Could you check a few things on this model? Use its own coordinates, in mm. Face numbers are marked on the shaded views. Give positions to 0.01 mm unless a question says otherwise; leave off trailing zeros. Order: outer loops, then holes, each group sorted by start corner. A loop starts at its lowest first (then second) coordinate and runs counter-clockwise, first axis right, second up. Notation, with made-up numbers: (-35.75, -13.5) -> (8.25, -13.5) arc R29 cw to (8.25, 8.5) -> close; hole circle Ø3 at (-22, 6.25). An arc over 180 degrees is marked (long way). One line per item, written item: value.
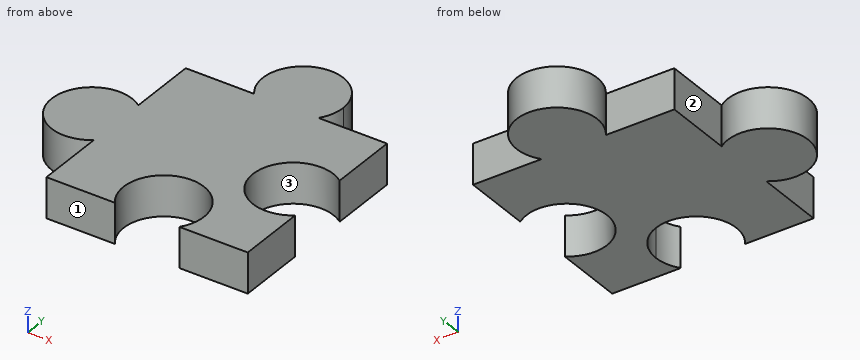
```python
from build123d import *

# Parameters (mm, degrees)
F1_DEPTH = 2.54


with BuildPart() as f1:
    # F0 (on Top) → F1 (new body)
    with BuildSketch(Plane.XY):
        with BuildLine():
            Line((-49.9644750565, 16.7031875085), (-49.9644750565, 20.7671875085))
            ThreePointArc((-49.9644750565, 20.7671875085), (-54.0284750565, 18.7351875085), (-49.9644750565, 16.7031875085))
        make_face()
        with BuildLine():
            ThreePointArc((-48.9484750565, 18.7351875085), (-49.2166299914, 19.8711100411), (-49.9644750565, 20.7671875085))
            Line((-49.9644750565, 20.7671875085), (-49.9644750565, 16.7031875085))
            ThreePointArc((-49.9644750565, 16.7031875085), (-49.2166299914, 17.599264976), (-48.9484750565, 18.7351875085))
        make_face()
        with BuildLine():
            Line((-45.6464750565, 25.0851875085), (-49.9644750565, 25.0851875085))
            Line((-49.9644750565, 25.0851875085), (-49.9644750565, 20.7671875085))
            ThreePointArc((-49.9644750565, 20.7671875085), (-49.2166299914, 19.8711100411), (-48.9484750565, 18.7351875085))
            ThreePointArc((-48.9484750565, 18.7351875085), (-49.2166299914, 17.599264976), (-49.9644750565, 16.7031875085))
            Line((-49.9644750565, 16.7031875085), (-49.9644750565, 12.3851875085))
            Line((-49.9644750565, 12.3851875085), (-45.6464750565, 12.3851875085))
            ThreePointArc((-45.6464750565, 12.3851875085), (-44.4176935822, 16.3188430856), (-41.0744750565, 13.9091875085))
            ThreePointArc((-41.0744750565, 13.9091875085), (-41.2048194795, 13.1059689828), (-41.5824750565, 12.3851875085))
            Line((-41.5824750565, 12.3851875085), (-37.2644750565, 12.3851875085))
            Line((-37.2644750565, 12.3851875085), (-37.2644750565, 16.7031875085))
            ThreePointArc((-37.2644750565, 16.7031875085), (-41.3284750565, 18.7351875085), (-37.2644750565, 20.7671875085))
            Line((-37.2644750565, 20.7671875085), (-37.2644750565, 25.0851875085))
            Line((-37.2644750565, 25.0851875085), (-41.5824750565, 25.0851875085))
            ThreePointArc((-41.5824750565, 25.0851875085), (-43.6144750565, 24.0691875085), (-45.6464750565, 25.0851875085))
        make_face()
        with BuildLine():
            Line((-41.5824750565, 25.0851875085), (-45.6464750565, 25.0851875085))
            ThreePointArc((-45.6464750565, 25.0851875085), (-43.6144750565, 24.0691875085), (-41.5824750565, 25.0851875085))
        make_face()
        with BuildLine():
            ThreePointArc((-41.0744750565, 26.6091875085), (-44.4176935822, 29.0188430856), (-45.6464750565, 25.0851875085))
            Line((-45.6464750565, 25.0851875085), (-41.5824750565, 25.0851875085))
            ThreePointArc((-41.5824750565, 25.0851875085), (-41.2048194795, 25.8059689828), (-41.0744750565, 26.6091875085))
        make_face()
    extrude(amount=F1_DEPTH)


solid = f1.part
```
1) Suppose I cut it at B-B, the plane x = -40. Write out the boundary of the cut face in (y, z).
Answer below:
outline: (12.39, 0) -> (16.5, 0) -> (16.5, 2.54) -> (12.39, 2.54) -> close; (20.97, 0) -> (25.09, 0) -> (25.09, 2.54) -> (20.97, 2.54) -> close
2) We'd pull the mould along Y, two halves only. Please class the marked faces 1, 2 and 3: +Y half, -Y half, draft (parallel to the pull), parting line (faces both ways), or undercut.
Answer below:
face 1: -Y half
face 2: draft
face 3: undercut
3) For P1, Ø1.3, axis at y = 22, z = 0.5, coming from the -X side; P2, Ø1.3, axis at x = -47.5, z = 1, coming from the +Y side; P3, Ø1, axis at x = -41.5, z = 1.5, coming from the +Y side; P4, Ø6, axis at x = -51.5, y = 26.5, coming from the +Z side, each with a flat end and sliding along its axis, tell me the tip position at first contact or that it passes through.
Answer below:
P1: stops at x = -49.96
P2: stops at y = 25.09
P3: stops at y = 28.57
P4: stops at z = 2.54
4) Suppose I cut it at D-D, the plane y = 27.5. Write out the boundary of the cut face in (x, z), then the cut area to 3 significant figures.
Answer below:
outline: (-45.99, 0) -> (-41.24, 0) -> (-41.24, 2.54) -> (-45.99, 2.54) -> close
area: 12.1 mm2
5) Suppose I cut it at C-C, the plane x = -48.5. Write out the boundary of the cut face in (y, z).
Answer below:
outline: (12.39, 0) -> (25.09, 0) -> (25.09, 2.54) -> (12.39, 2.54) -> close
6) Suppose I cut it at A-A, the plane z = 2. Write out the boundary of the cut face in (x, y).
Answer below:
outline: (-49.96, 12.39) -> (-45.65, 12.39) arc R2.54 cw (long way) to (-41.58, 12.39) -> (-37.26, 12.39) -> (-37.26, 16.7) arc R2.54 cw (long way) to (-37.26, 20.77) -> (-37.26, 25.09) -> (-41.58, 25.09) arc R2.54 ccw (long way) to (-45.65, 25.09) -> (-49.96, 25.09) -> (-49.96, 20.77) arc R2.54 ccw (long way) to (-49.96, 16.7) -> close
7) If I drill on line 1 along X through (y, z) = (14, 0.6); line 2 along X through (y, z) = (16.5, 0.6); line 3 along Y through (x, z) = (-46.5, 0.95), over which ranges is the centre line in solid material (lowest first)?
Answer below:
line 1: x = -49.96 to -46.15, -41.08 to -37.26
line 2: x = -52.69 to -50.28, -49.96 to -39.99, -37.58 to -37.26
line 3: y = 12.39 to 25.09
